Autodesk Inventor part; units mm, degrees
ref_plane "Work Plane1" through (17.549, 69.5929, -193.2) normal (0.2445129, 0.9696461, 0) x (0, 0, 1)
ref_plane "YZ Plane" through (0, 0, 0) normal (1, 0, 0) x (0, 1, 0)
ref_plane "XZ Plane" through (0, 0, 0) normal (0, 1, 0) x (-1, 0, 0)
sketch "Sketch1" plane through (0, 0, 0) normal (0, 1, 0) x (-1, 0, 0)
  line L0 (8, 0) -> (102.94, 0)
  line L1 (110.94, -8) -> (110.94, -185.2)
  line L2 (102.94, -193.2) -> (8, -193.2)
  line L3 (0, -185.2) -> (0, -8)
  circle A0 centre (86.7029, -32) radius 2.1
  circle A1 centre (88.297, -158.2) radius 2.1
  circle A2 centre (22.6, -158.501) radius 2.1
  circle A3 centre (21.4029, -32) radius 2.1
  arc A4 (110.94, -8) -> (102.94, 0) centre (102.94, -8) ccw
  arc A5 (8, 0) -> (0, -8) centre (8, -8) ccw
  arc A6 (0, -185.2) -> (8, -193.2) centre (8, -185.2) ccw
  arc A7 (102.94, -193.2) -> (110.94, -185.2) centre (102.94, -185.2) ccw
  point P0 (0, 0)
  dimension "d0" = 110.94
  dimension "d1" = 193.2
  dimension "d2" = 4.2
  dimension "d3" = 4.2
  dimension "d4" = 65.3
  dimension "d5" = 65.697
  dimension "d6" = 4.2
  dimension "d7" = 4.2
  dimension "d8" = 126.2
  dimension "d9" = 126.501
  dimension "d10" = 0
  dimension "d11" = 22.6
  dimension "d12" = 35
  dimension "d13" = 8
extrude "Extrusion1" add sketch "Sketch1" along normal blind 2
sketch "Sketch3" plane through (0, 2, 0) normal (0, 1, 0) x (1, 0, 0)
  line L0 (-91, 41) -> (-12, 41)
  line L1 (-12, 41) -> (-12, 146)
  line L2 (-12, 146) -> (-91, 146)
  line L3 (-99.94, 72) -> (-91, 72)
  line L4 (-91, 118.2) -> (-99.94, 118.2)
  line L5 (-99.94, 118.2) -> (-99.94, 72)
  circle A0 centre (-88.297, 158.2) radius 2.1
  circle A1 centre (-86.7029, 32) radius 2.1
  line L6 (-91, 146) -> (-91, 118.2)
  line L7 (-91, 72) -> (-91, 41)
  line L8 (-102.94, 0) -> (-8, 0)
  line L9 (0, 8) -> (0, 185.2)
  line L10 (-110.94, 185.2) -> (-110.94, 8)
  point P0 (0, 0)
  dimension "d22" = 105
  dimension "d26" = 40
  dimension "d27" = 40
  dimension "d32" = 12
  dimension "d33" = 41
  dimension "d34" = 11
  dimension "d35" = 79
  dimension "d36" = 79
extrude "Extrusion3" cut sketch "Sketch3" against normal blind 7.5 contours L7 L3 L5 L4 L6 L2 L1 L0
sketch "Sketch4" plane through (0, 2, 0) normal (0, 1, 0) x (1, 0, 0)
  line L0 (-91, 146) -> (-12, 146)
  line L1 (-12, 146) -> (-12, 41)
  line L2 (-12, 41) -> (-91, 41)
  line L3 (-91, 41) -> (-91, 72)
  line L4 (-91, 72) -> (-99.94, 72)
  line L5 (-99.94, 72) -> (-99.94, 118.2)
  line L6 (-99.94, 118.2) -> (-91, 118.2)
  line L7 (-91, 118.2) -> (-91, 146)
  line L8 (-8, 193.2) -> (-102.94, 193.2)
  arc A0 (-102.94, 193.2) -> (-110.94, 185.2) centre (-102.94, 185.2) ccw
  line L9 (-110.94, 185.2) -> (-110.94, 8)
  arc A1 (-110.94, 8) -> (-102.94, 0) centre (-102.94, 8) ccw
  line L10 (-102.94, 0) -> (-8, 0)
  arc A2 (-8, 0) -> (0, 8) centre (-8, 8) ccw
  line L11 (0, 8) -> (0, 185.2)
  arc A3 (0, 185.2) -> (-8, 193.2) centre (-8, 185.2) ccw
  circle A4 centre (-86.7029, 32) radius 2.1
  circle A5 centre (-88.297, 158.2) radius 2.1
  circle A6 centre (-22.6, 158.501) radius 2.1
  circle A7 centre (-21.4029, 32) radius 2.1
  arc A8 (-108.94, 8) -> (-102.94, 2) centre (-102.94, 8) ccw
  line L12 (-108.94, 8) -> (-108.94, 185.2)
  arc A9 (-102.94, 191.2) -> (-108.94, 185.2) centre (-102.94, 185.2) ccw
  line L13 (-102.94, 191.2) -> (-8, 191.2)
  arc A10 (-2, 185.2) -> (-8, 191.2) centre (-8, 185.2) ccw
  line L14 (-2, 185.2) -> (-2, 8)
  arc A11 (-8, 2) -> (-2, 8) centre (-8, 8) ccw
  line L15 (-8, 2) -> (-102.94, 2)
  point P0 (0, 0)
  dimension "d37" = 2
extrude "Extrusion4" add sketch "Sketch4" along normal blind 60 contours A3 L11 A2 L10 A1 L9 A0 L8
sketch "Sketch5" plane through (-102.94, 0, 0) normal (0, 0, 1) x (1, 0, 0)
  line L0 (-8, 0) -> (-8, 62)
  line L1 (-8, 14) -> (102.94, 62)
  line L2 (102.94, 0) -> (102.94, 62)
  line L3 (0, 0) -> (-8, 0)
  line L4 (0, 62) -> (-8, 62)
  line L5 (-8, 14) -> (-8, 62)
  line L6 (102.94, 62) -> (94.94, 62)
  line L7 (-8, 62) -> (102.94, 62)
  dimension "d40" = 14
  dimension "d41" = 0
extrude "Extrusion5" cut sketch "Sketch5" along normal mid plane 1000
sketch "Sketch6" plane through (-8, 0, -193.2) normal (0, 0, -1) x (-1, 0, 0)
  line L0 (102.94, 0) -> (102.94, 14)
  line L1 (102.94, 14) -> (-25.549, 69.5929)
  line L2 (94.94, 17.4613) -> (102.94, 14)
  line L3 (-25.549, 69.5929) -> (-8, 0)
  line L4 (0, 0) -> (-8, 0)
  line L5 (-8, 0) -> (0, 0)
  line L6 (0, 0) -> (0, 58.5387)
  line L7 (0, 0) -> (0, 58.5387)
  point P0 (-8, 62)
  dimension "d47" = 140
extrude "Extrusion6" add sketch "Sketch6" against normal blind 193.2
fillet "Fillet1" radius 8 2 edges at (8.7745, 34.7964, -193.2) (8.7745, 34.7964, 0)
ref_plane "Work Plane1" through (17.549, 69.5929, -193.2) normal (0.2445129, 0.9696461, 0) x (0, 0, 1)
sketch "Sketch9" plane through (17.549, 69.5929, -193.2) normal (0.2445129, 0.9696461, 0) x (0, 0, 1)
  line L0 (2, -22.0706) -> (191.2, -22.0706)
  line L1 (191.2, -100.3044) -> (191.2, -8.2462)
  line L2 (2, -22.0706) -> (191.2, -22.0706)
  line L3 (191.2, -22.0706) -> (191.2, -10)
  line L4 (183.2, -2) -> (10, -2)
  line L5 (2, -10) -> (2, -22.0706)
  line L6 (8, 0) -> (185.2, 0)
  arc A0 (191.2, -10) -> (183.2, -2) centre (183.2, -10) ccw
  arc A1 (10, -2) -> (2, -10) centre (10, -10) ccw
  point P0 (193.2, 0)
  point P1 (191.2, -2)
  dimension "d55" = 2
  dimension "d56" = 8
extrude "Extrusion7" cut sketch "Sketch9" against normal up to surface surface through (-55.47, 2, -96.6) normal (0, 1, 0)
sketch "Sketch10" plane through (-110.94, 14, -8) normal (-0.397092, 0.9177788, 0) x (0.9177788, 0.397092, 0)
  line L0 (8.7167, -6) -> (127.3869, -6)
  ellipse E0 centre (8.7167, 0) end of major axis (15.2542, 0) minor radius 6 (2.1792, 0) -> (8.7167, -6) ccw
  line L1 (2.1792, 177.2) -> (2.1792, 0)
  ellipse E1 centre (8.7167, 177.2) end of major axis (15.2542, 177.2) minor radius 6 (8.7167, 183.2) -> (2.1792, 177.2) ccw
  line L2 (127.3869, 183.2) -> (8.7167, 183.2)
  ellipse E2 centre (127.3869, 175.2) end of major axis (137.4774, 175.2) minor radius 8 (137.4774, 175.2) -> (127.3869, 183.2) ccw
  line L3 (137.4774, 175.2) -> (137.4774, 2)
  ellipse E3 centre (127.3869, 2) end of major axis (117.2964, 2) minor radius 8 (127.3869, -6) -> (137.4774, 2) ccw
  ellipse E4 centre (129.9095, 0) end of major axis (140, 0) minor radius 8 (129.9095, -8) -> (140, 0) ccw
  line L4 (140, 177.2) -> (140, 0)
  ellipse E5 centre (129.9095, 177.2) end of major axis (140, 177.2) minor radius 8 (140, 177.2) -> (129.9095, 185.2) ccw
  line L5 (8.7167, 185.2) -> (129.9095, 185.2)
  ellipse E6 centre (8.7167, 177.2) end of major axis (0, 177.2) minor radius 8 (8.7167, 185.2) -> (0, 177.2) ccw
  line L6 (0, 0) -> (0, 177.2)
  ellipse E7 centre (8.7167, 0) end of major axis (0, 0) minor radius 8 (0, 0) -> (8.7167, -8) ccw
  line L7 (129.9095, -8) -> (8.7167, -8)
  point P0 (96.2591, -8)
properties part number "Front"
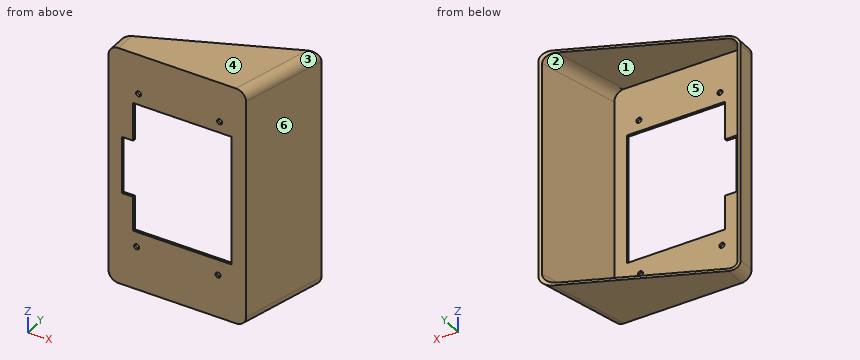
Geometry check sheet. Reference: the model listing, model coordinates, mm. Face numbers are marked on the shaded views. A direction names the side the tool comes from. Coordinates: 2 decimals unless noted, no trailing zeros. Loops run counter-clockwise (first coordinate to the right, second up) from the corner with the lowest first, then second, coordinate; pieces in that order, holes last.
Item 1: Sectioned sample at A-A, the plane z = -50. Record the boundary of the cut face in (x, y), then the cut area to 3 significant figures.
Item 2: Go/stop test with flat-tipped pins: pin 1 Ø6.5 at (y, z) = (11, -53.5) entering from +X; pin 2 Ø2.5 at (x, z) = (-22.6, -158.501) entering from -Y; pin 3 Ø2 at (y, z) = (1.5, -139) entering from +X. Record where each tip stops, or that it passes through.
Item 3: Sectioned sample at B-B, the plane x = -71. Record the boundary of the cut face in (y, z).
Item 4: Sectioned sample at C-C, the plane z = -12. Record the boundary of the cut face in (x, y).
Item 5: Access from +Z, -Z, +X, -X, +Y, -Y to the whole of each face (thin tool, end or side, straight path). Record for the marked faces 5 and 6.
Item 6: Thickness scan on line 1 (Z direction, x = -3, y = 28); line 2 (X direction, y = 1.2, z = -158.2); line 3 (Y direction, x = -100.5, z = -152). Record the ranges inside material, lowest first.
Item 7: Release check for a two-part mould opening along X. For the marked faces 1, 2, 3 and 4 record: released by +X, released by -X, zero draft, split by the parting line, or undercut.
Check result:
1. outline: (-110.94, 0) - (-91, 0) - (-91, 2) - (-108.94, 2) - (-108.94, 14.87) - (-110.94, 14) - close; (-12, 0) - (0, 0) - (17.55, 69.59) - (15.23, 68.59) - (-1.56, 2) - (-12, 2) - close
1. area: 228 mm2
2. pin 1: stops at x = 3.59
2. pin 2: passes through
2. pin 3: stops at x = 0.63
3. outline: (0, -193.2) - (31.28, -193.2) - (31.28, -191.2) - (2, -191.2) - (2, -146) - (0, -146) - close; (0, -41) - (2, -41) - (2, -2) - (31.28, -2) - (31.28, 0) - (0, 0) - close
4. outline: (-110.94, 0) - (0, 0) - (17.55, 69.59) - (15.23, 68.59) - (-1.56, 2) - (-108.94, 2) - (-108.94, 14.87) - (-110.94, 14) - close
5. face 5: +Y
5. face 6: +Z, -Z, +X, -Y
6. line 1: z = -193.2 to -191.2, -2 to 0
6. line 2: x = -110.94 to -90.4, -86.2 to -24.68, -20.52 to 0.3
6. line 3: y = 0 to 2
7. face 1: undercut
7. face 2: undercut
7. face 3: released by +X
7. face 4: zero draft
